Part model, mm, in its own coordinate system. Coordinates: 2 decimals unless noted, no trailing zeros. Write each loop counter-clockwise with the first axis right and the second up, starting at its lowest first coordinate (ties: lowest second). Pieces come first, ordered by that corner, then holes. Notation, with made-up numbers: (82, -39.75) - (127, -39.75) arc R20 cw to (127, -2.75) - close; hole circle Ø6 at (71, 65.25). An arc over 180 degrees is marked (long way). Use one line per item in the form item = value. Start each with the question number.
from build123d import *

# Parameters (mm, degrees)
SKETCH1_W               = 73.7
SKETCH1_H               = 65.6
BOSS_EXTRUDE1_DEPTH     = 2
FILLET1_R               = 1
CUT_EXTRUDE1_DEPTH      = 88.9202053
CUT_EXTRUDE1_DEPTH_BACK = 88.9202053
SKETCH2_R               = 1.6


with BuildPart() as part:
    # Sketch1 → Boss-Extrude1 (new body)
    with BuildSketch(Plane(origin=(0, 0, 0), x_dir=(0, 0, -1), z_dir=(1, 0, 0))):
        with Locations((0, -47)):
            Rectangle(SKETCH1_W, SKETCH1_H)
    extrude(amount=BOSS_EXTRUDE1_DEPTH)

    # Fillet1
    fillet1_edges = [part.edges().sort_by_distance(p)[0] for p in [
        (1, -14.2, 36.85),
        (1, -14.2, -36.85),
        (1, -79.8, -36.85),
        (1, -79.8, 36.85),
    ]]
    fillet(fillet1_edges, radius=FILLET1_R)

    # Sketch2 → Cut-Extrude1 (cut, two sides: drawn at the far end of the back side and taken through both)
    with BuildSketch(Plane(origin=(0, 0, 0), x_dir=(0, 0, -1), z_dir=(1, 0, 0)).offset(-CUT_EXTRUDE1_DEPTH_BACK)):
        with Locations((-32.6, -69.6)):
            Circle(SKETCH2_R)
        with Locations(Location((32.6, -69.6, 0), (0, 0, 180))):
            Circle(SKETCH2_R)
        with Locations((32.6, -24.4)):
            Circle(SKETCH2_R)
        with Locations(Location((-32.6, -24.4, 0), (0, 0, 180))):
            Circle(SKETCH2_R)
    extrude(amount=CUT_EXTRUDE1_DEPTH + CUT_EXTRUDE1_DEPTH_BACK, mode=Mode.SUBTRACT)


solid = part.part
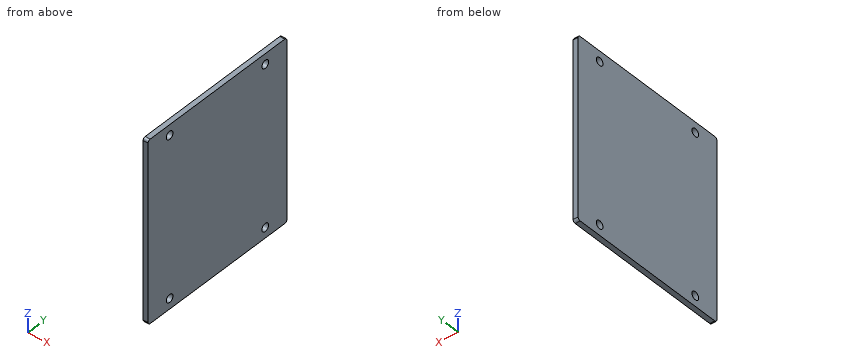
Q1. Drill centre lines: probe 1 along Y at (x, z) = (1, -32.6); probe 2 along Z at (x, y) = (0.85, -69.6); probe 3 along Z at (x, y) = (1.2, -23.5). Where is each one in solid material? Low to high.
Q2. Slice it at A-A (z = -32.6). List the corners of the cut face in (x, y).
Q3. Slice it at B-B (y = -24.4). List the corners of the cut face in (x, z), plus the area to 3 significant figures.
Solution:
q1.probe_1 = -79.8 to -71.2, -68 to -26, -22.8 to -14.2
q1.probe_2 = -36.85 to -34.2, -31 to 31, 34.2 to 36.85
q1.probe_3 = -36.85 to -33.92, -31.28 to 31.28, 33.92 to 36.85
q2.outline = (0, -79.8) - (2, -79.8) - (2, -71.2) - (0, -71.2) - close; (0, -68) - (2, -68) - (2, -26) - (0, -26) - close; (0, -22.8) - (2, -22.8) - (2, -14.2) - (0, -14.2) - close
q3.outline = (0, -36.85) - (2, -36.85) - (2, -34.2) - (0, -34.2) - close; (0, -31) - (2, -31) - (2, 31) - (0, 31) - close; (0, 34.2) - (2, 34.2) - (2, 36.85) - (0, 36.85) - close
q3.area = 135 mm2
